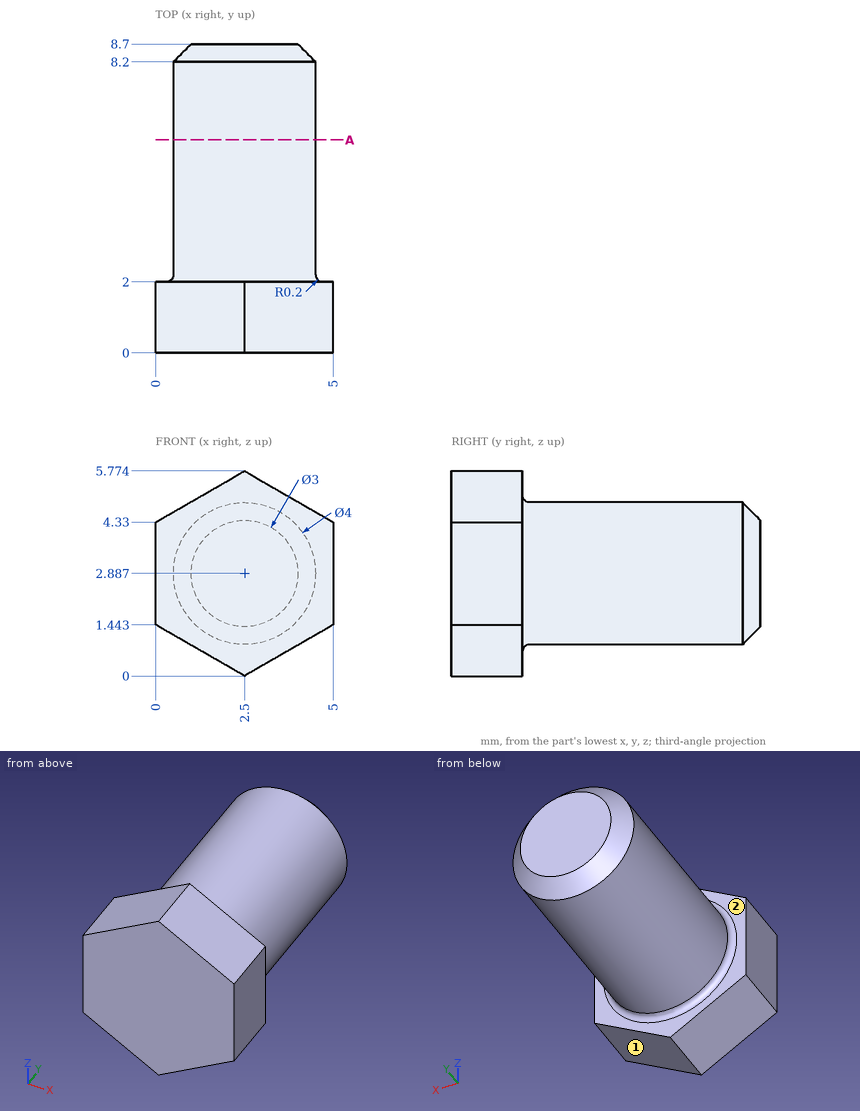
Here's the drawing with two shaded views (mm, measured from the low corner). I have some questions. A direction names the side the tool comes from. Give positions to 0.01 mm unless a question says otherwise; leave off trailing zeros. Order: outer loops, then holes, each group sorted by start corner. A loop starts at its lowest first (then second) coordinate and runs counter-clockwise, first axis right, second up. Notation, with made-up numbers: (-18, -5) -> (-8, -5) arc R18 cw to (-8, 15) -> close; hole circle Ø11 at (-24.5, -37). An arc over 180 degrees is marked (long way). One line per item, written item: value. Start each with the question number.
1. Imagine slicing it at A-A, the plane y = 6. List the corners of the cut face in (x, z) for me, plus the area to 3 significant figures.
2. I need wall thicknesses on probe 1 along Y at (x, z) = (3.95, 4.7); probe 2 along Z at (x, y) = (3.8, 4.5) (1 decimal); probe 3 along X at (y, z) = (3.5, 1.75) (1 decimal). Which ranges of each line are inside material? Lowest first, please. Write a range as from..to.
3. For the marked faces 1 and 2, which set-ups out of +Z, -Z, +X, -X, +Y, -Y let a thin tool reach every point of the face, with its end or its side?
Values follow:
1. outline: circle Ø4 at (2.5, 2.89)
1. area: 12.6 mm2
2. probe 1: y = 0..2
2. probe 2: z = 1.4..4.4
2. probe 3: x = 0.9..4.1
3. face 1: -Z, +X, +Y, -Y
3. face 2: +Y
